```python
from build123d import *

# Parameters (mm, degrees)
BOSS_EXTRUDE1_OUTLINE_R = 6.35
BOSS_EXTRUDE1_DEPTH     = 96.52


# Read off the part's stored shape, not the designer's step: Boss-Extrude1
with BuildPart() as part:
    # Boss-Extrude1 outline → Boss-Extrude1 (new body)
    with BuildSketch(Plane.XY.offset(-343.808229346)):
        with Locations((286.452894146, -18.033383804)):
            Circle(BOSS_EXTRUDE1_OUTLINE_R)
    extrude(amount=BOSS_EXTRUDE1_DEPTH)


solid = part.part
```
Check sheet for the modelled part. Datum: model origin and axes. Units: mm. Coordinates: 2 decimals unless noted, no trailing zeros. Loops run counter-clockwise (first coordinate to the right, second up) from the corner with the lowest first, then second, coordinate; pieces in that order, holes last.
1) Sectioned sample at B-B (x = 288.75). Record the boundary of the cut face in (y, z), and give its area (3 significant figures).
2) Material ranges on probe 1 along Y at (x, z) = (286.75, -295); probe 2 along Y at (x, z) = (288.25, -321.5); probe 3 along X at (y, z) = (-15.75, -283), recorded low to high.
3) Sectioned sample at C-C (y = -19.75). Record the boundary of the cut face in (x, z), and give its area (3 significant figures).
4) Gauge pin test, flat ends, axial feed: pin 1 (3 mm diameter, centred on y = -13, z = -327, fed in from +X); pin 2 (6 mm diameter, centred on x = 282, z = -295, fed in from +Y); pin 3 (2 mm diameter, centred on y = -16, z = -281, fed in from +X). Record the tip position at first contact, or that the pin passes through.
5) Sectioned sample at A-A (z = -319). Record the boundary of the cut face in (x, y), and give its area (3 significant figures).
Check sheet entries:
1. outline: (-23.95, -343.81) - (-12.11, -343.81) - (-12.11, -247.29) - (-23.95, -247.29) - close
1. area: 1,140 mm2
2. probe 1: y = -24.38 to -11.69
2. probe 2: y = -24.12 to -11.94
2. probe 3: x = 280.53 to 292.38
3. outline: (280.34, -343.81) - (292.57, -343.81) - (292.57, -247.29) - (280.34, -247.29) - close
3. area: 1,180 mm2
4. pin 1: stops at x = 291.73
4. pin 2: stops at y = -11.85
4. pin 3: stops at x = 292.72
5. outline: circle Ø12.7 at (286.45, -18.03)
5. area: 127 mm2
